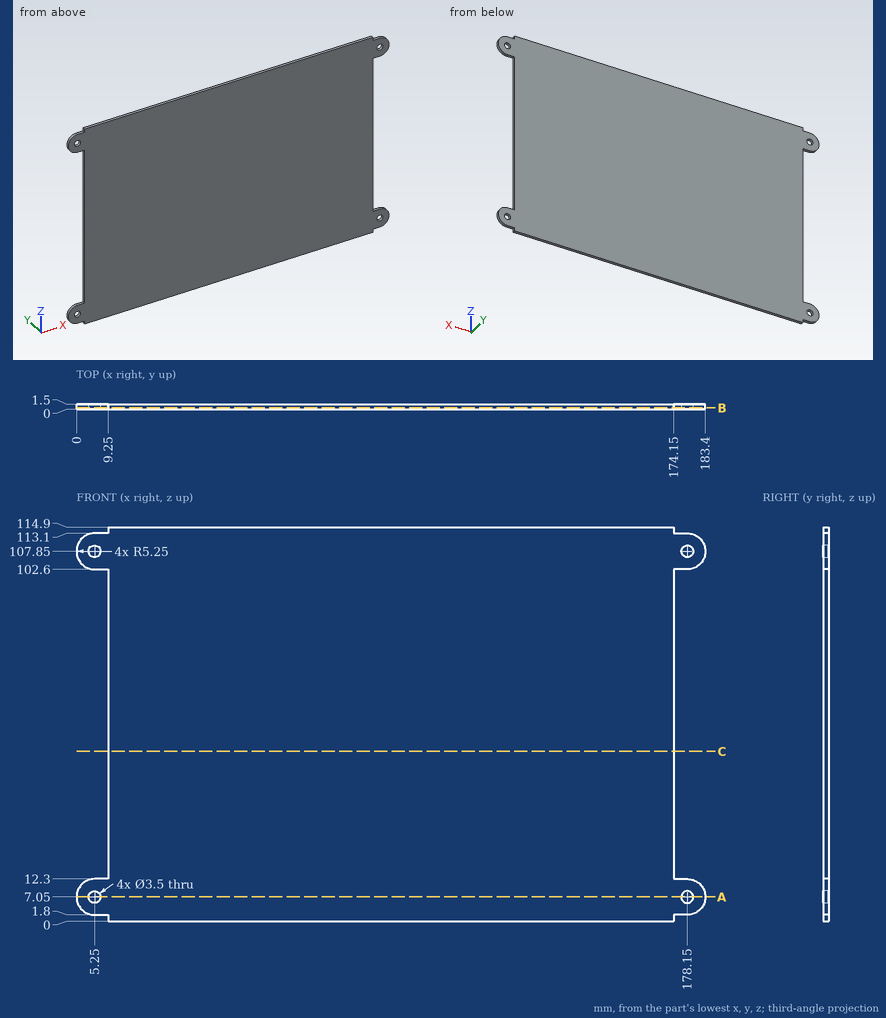
Source: three-view drawing plus pictorial views. Frame: mm from the lowest corner of the part. Coordinates: 2 decimals unless noted, no trailing zeros. Order: outer loops, then holes, each group sorted by start corner. A loop starts at its lowest first (then second) coordinate and runs counter-clockwise, first axis right, second up. Notation, with made-up numbers: M 68.5,33 L 88.5,33 A21 cw 88.5,53 Z; hole C 6.5,66 d11. An arc over 180 degrees is marked long. One line per question, with ' | ' between items.
Item 1: Section C-C (z = 49.5). Output: boundary loops of the cut face in (x, y), then the cut area to 3 significant figures.
Geometry results:
outline: M 9.25,0 L 174.15,0 L 174.15,1.5 L 9.25,1.5 Z | area: 247 mm^2
Item 2: Ray query, line 1 along Z through (x, y) = (5.25, 0.85); line 2 along X through (y, z) = (0.75, 7.05); line 3 along X through (y, z) = (0.1, 83). Return the intervals inside material, ascending.
Geometry results:
line 1: z = 1.8 to 5.3, 8.8 to 12.3, 102.6 to 106.1, 109.6 to 113.1 | line 2: x = 0 to 3.5, 7 to 176.4, 179.9 to 183.4 | line 3: x = 9.25 to 174.15
Item 3: Pin query (flat end, axial travel): pin 1 (2 mm diameter, centred on x = 5.25, z = 107.85, fed in from -Y); pin 2 (0.8 mm diameter, centred on x = 7, y = 1, fed in from +Z). Return the tip coordinate at first contact, or that it passes through.
Geometry results:
pin 1: passes through | pin 2: stops at z = 113.1
Item 4: Section B-B (y = 0.4). Output: boundary loops of the cut face in (x, z), then the cut area to 3 significant figures.
Geometry results:
outline: M 5.25,1.8 L 9.25,1.8 L 9.25,0 L 174.15,0 L 174.15,1.8 L 178.15,1.8 A5.25 ccw 178.15,12.3 L 174.15,12.3 L 174.15,102.6 L 178.15,102.6 A5.25 ccw 178.15,113.1 L 174.15,113.1 L 174.15,114.9 L 9.25,114.9 L 9.25,113.1 L 5.25,113.1 A5.25 ccw 5.25,102.6 L 9.25,102.6 L 9.25,12.3 L 5.25,12.3 A5.25 ccw Z; hole C 5.25,7.05 d3.5; hole C 5.25,107.85 d3.5; hole C 178.15,7.05 d3.5; hole C 178.15,107.85 d3.5 | area: 19,200 mm^2
Item 5: Section A-A (z = 7.05). Output: boundary loops of the cut face in (x, y), then the cut area to 3 significant figures.
Geometry results:
outline: M 0,0 L 3.5,0 L 3.5,1.5 L 0,1.5 Z; M 7,0 L 176.4,0 L 176.4,1.5 L 7,1.5 Z; M 179.9,0 L 183.4,0 L 183.4,1.5 L 179.9,1.5 Z | area: 265 mm^2
